from build123d import *

# Parameters (mm, degrees)
SKETCH1_W           = 1299.221386713
SKETCH1_H           = 762
BOSS_EXTRUDE2_DEPTH = 508
SKETCH3_R           = 90.110640619
BOSS_EXTRUDE4_DEPTH = 762
SKETCH4_R           = 66.065626011
CUT_EXTRUDE1_DEPTH  = 1590.554721201
CHAMFER3_SIZE       = 12.7
SKETCH5_W           = 305.335237322
SKETCH5_H           = 167.392745924
CUT_EXTRUDE2_DEPTH  = 127
FILLET3_R           = 50.8


with BuildPart() as part:
    # Sketch1 → Boss-Extrude2 (new body)
    with BuildSketch(Plane(origin=(0, 0, 0), x_dir=(1, 0, 0), z_dir=(0, 1, 0))):
        with Locations((649.610693357, -381)):
            Rectangle(SKETCH1_W, SKETCH1_H)
    extrude(amount=BOSS_EXTRUDE2_DEPTH)

    # Sketch3 → Boss-Extrude4 (add, through all)
    with BuildSketch(Plane.XY.offset(762)):
        with Locations((199.400638449, 376.804670273)):
            Circle(SKETCH3_R)
    extrude(amount=-BOSS_EXTRUDE4_DEPTH)

    # Sketch4 → Cut-Extrude1 (cut, through all)
    with BuildSketch(Plane.XY.offset(762)):
        with Locations((245.395602091, 385.783170349)):
            Circle(SKETCH4_R)
    extrude(amount=-CUT_EXTRUDE1_DEPTH, mode=Mode.SUBTRACT)

    # Chamfer3
    chamfer3_edges = [part.edges().sort_by_distance(p)[0] for p in [
        (179.329976081, 385.783170349, 0),
        (179.329976081, 385.783170349, 762),
    ]]
    chamfer(chamfer3_edges, length=CHAMFER3_SIZE)

    # Sketch5 → Cut-Extrude2 (cut)
    with BuildSketch(Plane.XY.offset(762)):
        with Locations((1146.553768052, 83.696372962)):
            Rectangle(SKETCH5_W, SKETCH5_H)
    extrude(amount=-CUT_EXTRUDE2_DEPTH, mode=Mode.SUBTRACT)

    # Fillet3
    fillet3_edges = [part.edges().sort_by_distance(p)[0] for p in [
        (993.886149391, 83.696372962, 635),
    ]]
    fillet(fillet3_edges, radius=FILLET3_R)


solid = part.part
Design review of the part built by this model. Coordinates are the model's own, in mm. A direction names the side the tool comes from. Round coordinates to 2 decimals unless told otherwise and drop trailing zeros. Order: outer loops, then holes, each group sorted by start corner. A loop starts at its lowest first (then second) coordinate and runs counter-clockwise, first axis right, second up.
1) Consider section C-C (z = 567.5). State the section outline as (x, y) points, plus the area to 3 significant figures.
The answers:
outline: (0, 0) - (1299.22, 0) - (1299.22, 508) - (0, 508) - close; hole circle Ø132.13 at (245.4, 385.78)
area: 646,000 mm2
2) Clearance check with a flat-ended pin moving along its axis: pin 1 Ø10 at (x, z) = (1131, 641.5) entering from -Y. State where the tip first meets the part, or that it passes through.
The answers:
pin 1: stops at y = 167.39
3) Consider section A-A (y = 113.5). State the section outline as (x, z) points, plus the area to 3 significant figures.
The answers:
outline: (0, 0) - (1299.22, 0) - (1299.22, 635) - (1044.69, 635) arc R50.8 cw to (993.89, 685.8) - (993.89, 762) - (0, 762) - close
area: 952,000 mm2
4) For L1, parallel to X at y = 349, z = 644; L2, parallel to X at y = 437.5, z = 331; L3, parallel to Z at x = 1098, y = 99, list the stretches that pass through material, from the lowest coordinate up.
The answers:
L1: x = 0 to 190.52, 300.27 to 1299.22
L2: x = 0 to 204.29, 286.51 to 1299.22
L3: z = 0 to 635
5) Consider section B-B (x = 1102.5). State the section outline as (y, z) points, plus the area to 3 significant figures.
The answers:
outline: (0, 0) - (508, 0) - (508, 762) - (167.39, 762) - (167.39, 635) - (0, 635) - close
area: 366,000 mm2
6) Draft analysis for pull direction X (two halves, no side actions). For faces 1 (the cylindrical face through (1008.37, 84.87, 650.28)), 2 (the conical face through (276.17, 326.62, 749.92)), 3 (the flat face through (641, 250, 0)), 4 (the cylindrical face through (236.795, 451.287, 386.156)), state which applies: released by +X, released by -X, zero draft, split by the parting line, or undercut.
The answers:
face 1: released by +X
face 2: undercut
face 3: zero draft
face 4: undercut
7) Machinability: for faces 5 (the flat face through (993.886, 83, 724)), 6 (the flat face through (641, 508, 376)), which of the approach directions +Z, -Z, +X, -X, +Y, -Y give a long, thin tool a straight path to every point of the face, cutting with its end or side? Answer none if there is none.
The answers:
face 5: +Z, +X, -Y
face 6: +Z, -Z, +X, -X, +Y
